Can you work these out from the drawing? Everything is in mm from the part's minimum corner. Coordinates: 2 decimals unless noted, no trailing zeros. Write each loop counter-clockwise with the first axis right and the second up, starting at its lowest first coordinate (ties: lowest second). Pieces come first, ordered by that corner, then holes.
(1) Imagine slicing it at B-B, the plane y = 100.5. List the corners of the cut face in (x, z) for me, plus the area to 3 significant figures.
(2) Imagine slicing it at A-A, the plane x = 162. List the corners of the cut face in (y, z) for me.
(3) Thinking about a two-plate mould opening in X: for the marked faces 1, 2 and 3, which applies, released by +X, released by -X, zero draft, split by the parting line, or undercut?
(4) Imagine slicing it at C-C, the plane z = 31. List the corners of the cut face in (x, y) for me.
(5) Please list where these lines run through material, in increasing order: probe 1 along Z at (x, y) = (138, 60.5); probe 2 along Y at (x, z) = (38, 47).
(6) For pin 1 Ø7.5 at (x, z) = (83.5, 34.5) entering from -Y, with a flat end and sliding along its axis, tell me the tip position at first contact or that it passes through.
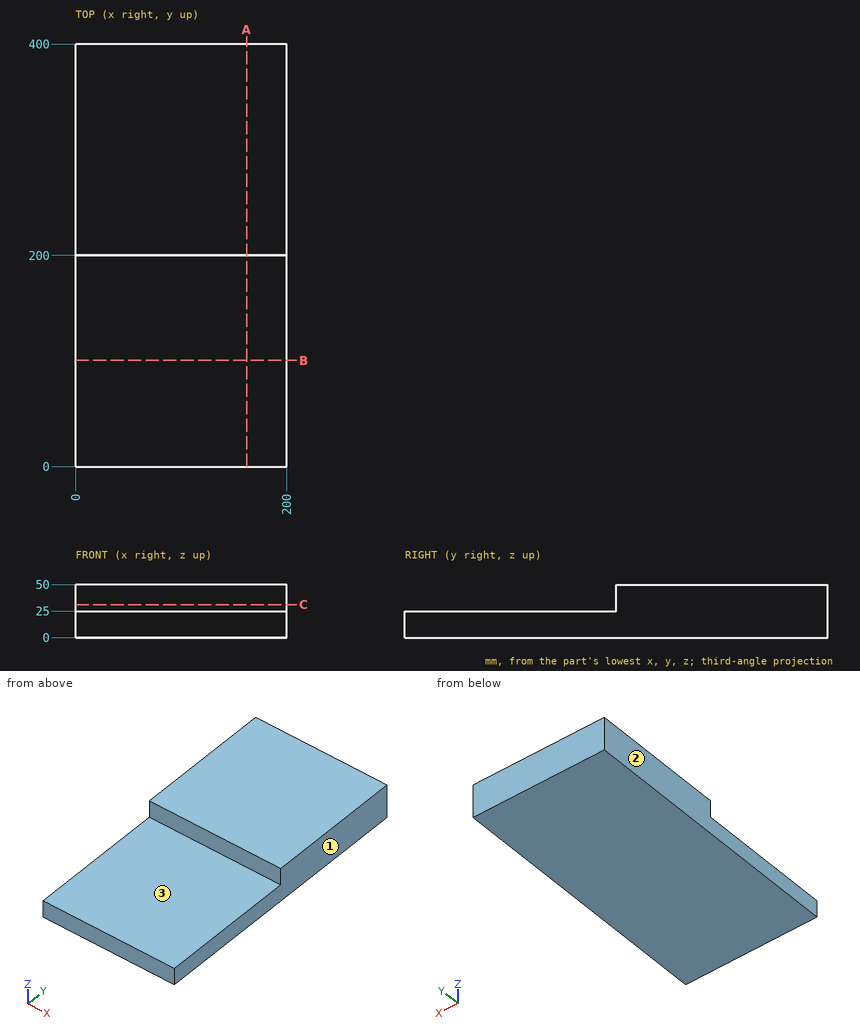
Recorded:
1. outline: (0, 0) - (200, 0) - (200, 25) - (0, 25) - close
1. area: 5,000 mm2
2. outline: (0, 0) - (400, 0) - (400, 50) - (200, 50) - (200, 25) - (0, 25) - close
3. face 1: released by +X
3. face 2: released by -X
3. face 3: zero draft
4. outline: (0, 200) - (200, 200) - (200, 400) - (0, 400) - close
5. probe 1: z = 0 to 25
5. probe 2: y = 200 to 400
6. pin 1: stops at y = 200
